from build123d import *

# Parameters (mm, degrees)
SKETCH1_W           = 371.348752766
SKETCH1_H           = 757.75300928
SKETCH1_W_2         = 369.177102164
BOSS_EXTRUDE2_DEPTH = 400
SKETCH2_W           = 762.063158907
SKETCH2_H           = 50
BOSS_EXTRUDE3_DEPTH = 761
SKETCH3_W           = 800
SKETCH3_H           = 756.769192836
CUT_EXTRUDE1_DEPTH  = 20
SKETCH4_W           = 240.999510027
SKETCH4_H           = 373.99553593
CUT_EXTRUDE2_DEPTH  = 164
SKETCH5_W           = 366.749799027
SKETCH5_H           = 332.09627471
CUT_EXTRUDE4_DEPTH  = 29
SKETCH6_W           = 240.999510027
SKETCH6_H           = 373.99553593
CUT_EXTRUDE5_DEPTH  = 29
SKETCH7_W           = 372.210354375
SKETCH7_H           = 328.047679772
CUT_EXTRUDE7_DEPTH  = 29
CHAMFER2_SIZE       = 10


with BuildPart() as part:
    # Sketch1 → Boss-Extrude2 (new body)
    with BuildSketch(Plane.XY):
        Polygon((-56.757111626, 778.097101449), (-56.757111626, -21.902898551), (743.242888374, -21.902898551), (743.242888374, 778.097101449), (475.242888374, 978.097101449), (209.242888374, 978.097101449), align=None)
        with Locations((147.788525051, 378.87650464)):
            Rectangle(SKETCH1_W, SKETCH1_H, mode=Mode.SUBTRACT)
        with Locations((539.588756493, 378.87650464)):
            Rectangle(SKETCH1_W_2, SKETCH1_H, mode=Mode.SUBTRACT)
    extrude(amount=BOSS_EXTRUDE2_DEPTH)

    # Sketch2 → Boss-Extrude3 (add)
    with BuildSketch(Plane(origin=(0, 0, 0), x_dir=(1, 0, 0), z_dir=(0, 1, 0))):
        with Locations((343.145728122, -25)):
            Rectangle(SKETCH2_W, SKETCH2_H)
    extrude(amount=BOSS_EXTRUDE3_DEPTH)

    # Sketch3 → Cut-Extrude1 (cut)
    with BuildSketch(Plane.XY.offset(400)):
        with Locations((343.242888374, 378.384596418)):
            Rectangle(SKETCH3_W, SKETCH3_H)
    extrude(amount=-CUT_EXTRUDE1_DEPTH, mode=Mode.SUBTRACT)

    # Sketch4 → Cut-Extrude2 (cut)
    with BuildSketch(Plane(origin=(0, 978.097101449, 0), x_dir=(1, 0, 0), z_dir=(0, 1, 0))):
        with Locations((343.242888374, -199.553704611)):
            Rectangle(SKETCH4_W, SKETCH4_H)
    extrude(amount=-CUT_EXTRUDE2_DEPTH, mode=Mode.SUBTRACT)

    # Sketch5 → Cut-Extrude4 (cut)
    with BuildSketch(Plane.XZ.offset(-757.75300928)):
        with Locations((148.316814088, 212.995071619)):
            Rectangle(SKETCH5_W, SKETCH5_H)
    extrude(amount=-CUT_EXTRUDE4_DEPTH, mode=Mode.SUBTRACT)

    # Sketch6 → Cut-Extrude5 (cut)
    with BuildSketch(Plane(origin=(0, 814.097101449, 0), x_dir=(1, 0, 0), z_dir=(0, 1, 0))):
        with Locations((343.242888374, -199.553704611)):
            Rectangle(SKETCH6_W, SKETCH6_H)
    extrude(amount=-CUT_EXTRUDE5_DEPTH, mode=Mode.SUBTRACT)

    # Sketch7 → Cut-Extrude7 (cut)
    with BuildSketch(Plane.XZ.offset(-757.75300928)):
        with Locations((540.059154896, 214.239949558)):
            Rectangle(SKETCH7_W, SKETCH7_H)
    extrude(amount=-CUT_EXTRUDE7_DEPTH, mode=Mode.SUBTRACT)

    # Chamfer2
    chamfer2_edges = [part.edges().sort_by_distance(p)[0] for p in [
        (343.242888374, 785.097101449, 12.555936646),
        (331.691713601, 785.097101449, 212.995071619),
        (353.953977708, 785.097101449, 214.239949558),
    ]]
    chamfer(chamfer2_edges, length=CHAMFER2_SIZE)


solid = part.part
Source: CAD feature listing. Evaluate the final solid. Frame: model axes, mm. A direction names the side the tool comes from. Coordinates: 2 decimals unless noted, no trailing zeros. Loops run counter-clockwise (first coordinate to the right, second up) from the corner with the lowest first, then second, coordinate; pieces in that order, holes last. Notation, with made-up numbers: (88.5, 59.5) - (146.5, 59.5) arc R16 cw to (146.5, 65.5) - close; hole circle Ø10 at (69.25, -18.75). An arc over 180 degrees is marked (long way). One line per question, with ' | ' between items.
1) First-contact query: P1, Ø0.6, axis at x = 725.5, z = 164, coming from the +Y side; P2, Ø5.5, axis at x = 735, y = 326.5, coming from the +Z side; P3, Ø0.9, axis at x = 130.5, z = 48, coming from the +Y side; P4, Ø8, axis at x = 72.5, y = 88, coming from the -Z side. Flat tips, straight axial feed; report the tip coordinate or a pass-through.
Report:
P1: stops at y = 791.56 | P2: stops at z = 380 | P3: stops at y = 919.23 | P4: stops at z = 0
2) Section C-C, the plane z = 164.5. Return loops of the section in (x, y).
Report:
outline: (-56.76, -21.9) - (743.24, -21.9) - (743.24, 778.1) - (475.24, 978.1) - (463.74, 978.1) - (463.74, 786.75) - (726.16, 786.75) - (726.16, 757.75) - (724.18, 757.75) - (724.18, 0) - (355, 0) - (355, 757.75) - (353.95, 757.75) - (353.95, 775.1) - (343.95, 785.1) - (341.69, 785.1) - (331.69, 775.1) - (331.69, 757.75) - (333.46, 757.75) - (333.46, 0) - (-37.89, 0) - (-37.89, 757.75) - (-35.06, 757.75) - (-35.06, 786.75) - (222.74, 786.75) - (222.74, 978.1) - (209.24, 978.1) - (-56.76, 778.1) - close
3) Pull-direction query (Y, two-part tool) for faces 1 (the face through (342, 888, 12.556)), 2 (the face through (611.119, 876.697, 197.2)), 3 (the face through (537, 757.753, 389)); classes: released by +Y, released by -Y, zero draft, split by the parting line, or undercut.
Report:
face 1: zero draft | face 2: released by +Y | face 3: undercut
4) Section D-D, the plane y = 898. Return loops of the section in (x, z), then the cut area to 3 significant figures.
Report:
outline: (102.71, 0) - (582.57, 0) - (582.57, 400) - (102.71, 400) - close; hole (222.74, 12.56) - (463.74, 12.56) - (463.74, 386.55) - (222.74, 386.55) - close | area: 102,000 mm²
5) Set-up query: faces 4 (the face through (532, 772, 50.216)), 5 (the face through (249, 0, 227)), 6 (the face through (344, 384, 380)). Return all of +Z, -Z, +X, -X, +Y, -Y with unobstructed straight access to the full face (end or side cutting, diameter ignored); none if empty.
Report:
face 4: none | face 5: +Z | face 6: +Z, +X, -X
6) Section B-B, the plane y = 684.5. Return loops of the section in (x, z).
Report:
outline: (-56.76, 0) - (743.24, 0) - (743.24, 380) - (724.18, 380) - (724.18, 50) - (355, 50) - (355, 380) - (333.46, 380) - (333.46, 50) - (-37.89, 50) - (-37.89, 380) - (-56.76, 380) - close
7) Line query: line 1 along X through (y, z) = (470, 209.5); line 2 along Y through (x, z) = (212.5, 288); line 3 along Z through (x, y) = (352, 910.5). Output: solid intervals per line, ascending.
Report:
line 1: x = -56.76 to -37.89, 333.46 to 355, 724.18 to 743.24 | line 2: y = -21.9 to 0, 786.75 to 978.1 | line 3: z = 0 to 12.56, 386.55 to 400
8) Section A-A, the plane x = 376.5. Return loops of the section in (y, z).
Report:
outline: (-21.9, 0) - (978.1, 0) - (978.1, 12.56) - (795.1, 12.56) - (785.1, 22.56) - (785.1, 50.22) - (757.75, 50.22) - (757.75, 50) - (0, 50) - (0, 400) - (-21.9, 400) - close; (757.75, 378.26) - (785.1, 378.26) - (785.1, 386.55) - (978.1, 386.55) - (978.1, 400) - (757.75, 400) - close
